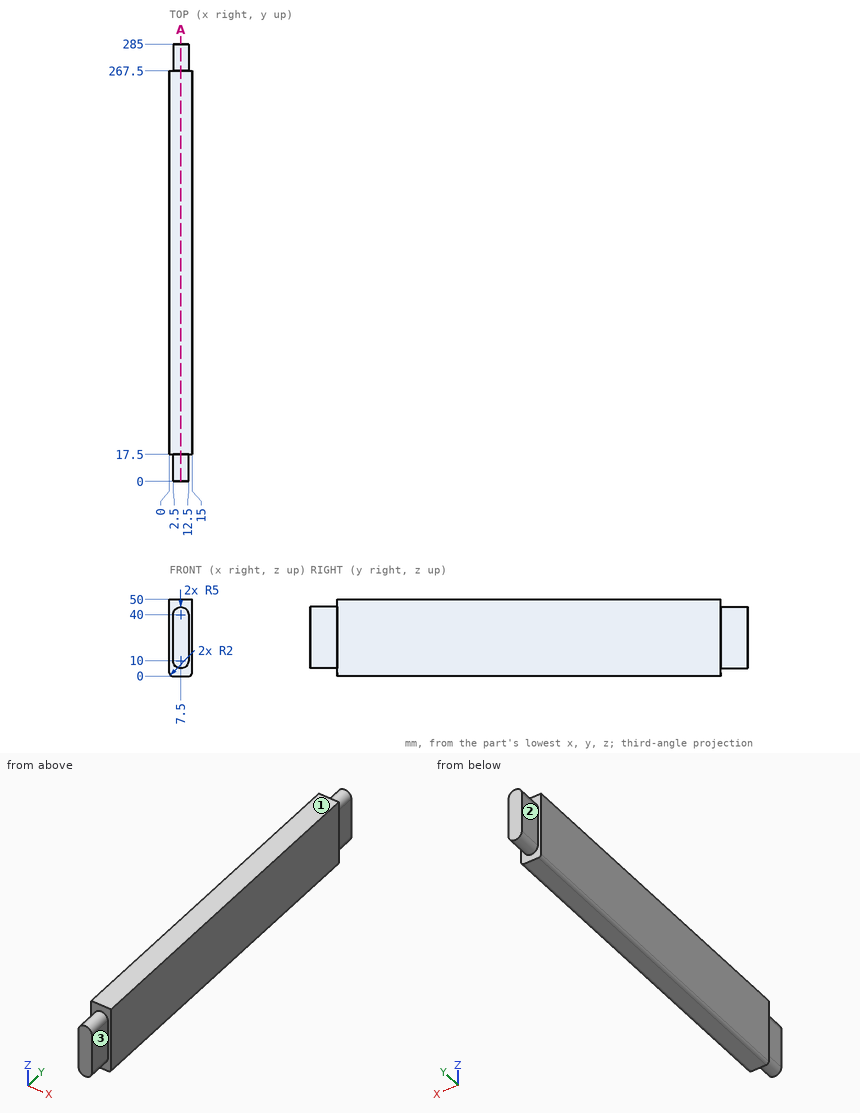
Design review of the part shown in the three views and the two pictorial views. Dimensions are in mm from the part's minimum x, y and z. A direction names the side the tool comes from. Round coordinates to 2 decimals unless told otherwise and drop trailing zeros. Loops run counter-clockwise (first coordinate to the right, second up) from the corner with the lowest first, then second, coordinate; pieces in that order, holes last. Notation, with made-up numbers: M 29,-28 L 79,-28 A31 cw 79,8 Z; hole C 44.25,78.25 d1. An arc over 180 degrees is marked long. Answer as a JSON object with one key per item and string values.
Item 1: Clearance check with flat-ended pins moving along their axes: P1, Ø5, axis at y = 273.5, z = 23.5, coming from the -X side; P2, Ø5, axis at y = 10.5, z = 30, coming from the +X side. State where each tip first meets the part, or that it passes through.
Answer sheet:
{"P1": "stops at x = 2.5", "P2": "stops at x = 12.5"}
Item 2: Machinability: for the marked faces 1, 2 and 3, which of the approach directions +Z, -Z, +X, -X, +Y, -Y give a long, thin tool a straight path to every point of the face, cutting with its end or side? Answer none if there is none.
Answer sheet:
{"face 1": "+Z, +X, -X, +Y, -Y", "face 2": "+Z, -Z, -X, +Y", "face 3": "+Z, -Z, +X, -Y"}
Item 3: Wall thickness on L1, parallel to Y at x = 11.5, z = 48: over which ranges is the line inside the solid? List them lowest first. Write a range as from..to.
Answer sheet:
{"L1": "y = 17.5..267.5"}
Item 4: We need section A-A on x = 7.5. Give the boundary of the cut face in (y, z), and give its area (3 significant figures).
Answer sheet:
{"outline": "M 0,5 L 17.5,5 L 17.5,0 L 267.5,0 L 267.5,5 L 285,5 L 285,45 L 267.5,45 L 267.5,50 L 17.5,50 L 17.5,45 L 0,45 Z", "area": "13,900 mm^2"}
